from build123d import *

# Parameters (mm, degrees)
F1_DEPTH = 3.82
F2_R     = 2


with BuildPart() as f1:
    # F0 (on Right) → F1 (new body)
    with BuildSketch(Plane.YZ):
        Polygon((33.298553, -6.72), (33.298553, 8), (-61.701447, 8), (-96.385158, -15.782844), (-86.385158, -15.782844), (-61.701447, 0), align=None)
    extrude(amount=F1_DEPTH)

    # F2
    f2_edges = [f1.edges().sort_by_distance(p)[0] for p in [
        (0, -14.201447, 8),
        (0, -14.201447, -3.36),
        (0, -79.043303, -3.891422),
        (0, -74.043303, -7.891422),
        (0, -91.385158, -15.782844),
        (1.91, -61.701447, 0),
        (1.91, -86.385158, -15.782844),
    ]]
    fillet(f2_edges, radius=F2_R)


solid = f1.part
Model file for the job. Use its own axes, mm. A direction names the side the tool comes from. Coordinates: 2 decimals unless noted, no trailing zeros. Write each loop counter-clockwise with the first axis right and the second up, starting at its lowest first coordinate (ties: lowest second). Pieces come first, ordered by that corner, then holes. Notation, with made-up numbers: (-10, -20.5) -> (47, -20.5) arc R16 cw to (47, 9.5) -> close; hole circle Ø9 at (27, 58). An arc over 180 degrees is marked (long way). One line per item, written item: value. Start each with the question number.
1) Slice it at A-A on x = 2.65. Write the cut outline in (y, z), then the cut area to 3 significant figures.
2) Probe probe 1 along Y at (x, z) = (1.35, 6.75); probe 2 along Y at (x, z) = (2.4, -12.5); probe 3 along Z at (x, y) = (2.6, -86.5). List the from-to ranges inside material, lowest first.
3) Which spindle directions (+Z, -Z, +X, -X, +Y, -Y) get a long thin tool onto all of the face, cutting with end or side? Do faces 1 (the face through (2.897, -14.532, -3.337)), 2 (the face through (3.82, -18, 2)), 3 (the face through (0.601, -74.218, -7.326)). Say none if no direction does.
4) Pull direction Y, two halves, no side cores. Call faces 4 (the face through (2.897, -74.241, -8.018)), 5 (the face through (0.6, -78.96, -4.53)), 6 (the face through (0, -15, 1)): +Y half, -Y half, draft (parallel to the pull), parting line (faces both ways), or undercut.
5) Flat gauge pin, fed straight in: pin 1 Ø2 at (x, z) = (3.5, -10) entering from -Y. Where does the tip first touch, or does it go through?
Answers follow:
1. outline: (-96.39, -15.78) -> (-86.97, -15.78) arc R2 ccw to (-85.89, -15.47) -> (-62.26, -0.36) arc R2 cw to (-61.04, -0.05) -> (33.3, -6.72) -> (33.3, 8) -> (-61.7, 8) -> close
1. area: 1,300 mm2
2. probe 1: -63.33 to 33.3
2. probe 2: -91.6 to -81.25
2. probe 3: -15.73 to -9
3. face 1: -Z, +X, -X
3. face 2: +Z, -Z, +X, +Y, -Y
3. face 3: -Z, -X
4. face 4: undercut
4. face 5: -Y half
4. face 6: draft
5. pin 1: y = -89.41
